```python
from build123d import *

# Parameters (mm, degrees)
BOSS_EXTRUDE1_START             = 3.5
SKETCH1_W                       = 116
SKETCH1_H                       = 42
BOSS_EXTRUDE1_DEPTH             = 3.5
BOSS_EXTRUDE2_REACH             = 64.081
SKETCH2_R                       = 1.75
BOSS_EXTRUDE2_DIRECTION_2_REACH = 64.081
SKETCH2_3_R                     = 1.75
CUT_EXTRUDE1_DEPTH              = 54
BOSS_EXTRUDE3_DEPTH             = 25
BOSS_EXTRUDE5_START             = -4
SKETCH4_R                       = 1.5
BOSS_EXTRUDE5_DEPTH             = 4
SKETCH5_R                       = 1.5
BOSS_EXTRUDE6_DEPTH             = 4
FILLET1_R                       = 5
FILLET2_R                       = 1
SKETCH6_W                       = 116
SKETCH6_H                       = 71
BOSS_EXTRUDE7_DEPTH             = 4
SKETCH7_R                       = 1.5
BOSS_EXTRUDE8_DEPTH             = 4
LPATTERN1_COUNT                 = 2
LPATTERN1_PITCH                 = 112
FILLET3_R                       = 4


with BuildPart() as part:
    # Sketch1 → Boss-Extrude1 (new body)
    with BuildSketch(Plane(origin=(0, 0, 0), x_dir=(1, 0, 0), z_dir=(0, 1, 0)).offset(BOSS_EXTRUDE1_START)):
        Rectangle(SKETCH1_W, SKETCH1_H)
    extrude(amount=BOSS_EXTRUDE1_DEPTH)

    # Boss-Extrude2: up to this face of the body (flat: up to its plane)
    boss_extrude2_end = Plane(part.part.faces().sort_by_distance((58, 5.25, 0))[0])
    # Sketch2 → Boss-Extrude2 (add, up to the picked face)
    with BuildSketch(Plane(origin=(0, 0, 0), x_dir=(0, 0, -1), z_dir=(1, 0, 0)), mode=Mode.PRIVATE) as boss_extrude2_sk1:
        with BuildLine():
            ThreePointArc((10, 13), (8.586149806, 9.094875162), (5, 7))
            Line((5, 7), (10, 7))
            Line((10, 7), (21, 7))
            Line((21, 7), (21, 18))
            Line((21, 18), (15, 18))
            ThreePointArc((15, 18), (11.464466094, 16.535533906), (10, 13))
        make_face()
        with Locations(Location((15.5, 12.475, 0), (0, 0, 180))):
            Circle(SKETCH2_R, mode=Mode.SUBTRACT)
    boss_extrude2_tool1 = split(extrude(boss_extrude2_sk1.sketch, amount=BOSS_EXTRUDE2_REACH, mode=Mode.PRIVATE), bisect_by=boss_extrude2_end, keep=Keep.BOTH, mode=Mode.PRIVATE)
    # Sketch2 → Boss-Extrude2 (add, up to the picked face)
    with BuildSketch(Plane(origin=(0, 0, 0), x_dir=(0, 0, -1), z_dir=(1, 0, 0)), mode=Mode.PRIVATE) as boss_extrude2_sk2:
        with BuildLine():
            Line((-21, 18), (-21, 7))
            Line((-21, 7), (-5, 7))
            ThreePointArc((-5, 7), (-8.586149806, 9.094875162), (-10, 13))
            ThreePointArc((-10, 13), (-11.464466094, 16.535533906), (-15, 18))
            Line((-15, 18), (-21, 18))
        make_face()
        with Locations(Location((-15.5, 12.475, 0), (0, 0, 180))):
            Circle(SKETCH2_R, mode=Mode.SUBTRACT)
    boss_extrude2_tool2 = split(extrude(boss_extrude2_sk2.sketch, amount=BOSS_EXTRUDE2_REACH, mode=Mode.PRIVATE), bisect_by=boss_extrude2_end, keep=Keep.BOTH, mode=Mode.PRIVATE)
    add(boss_extrude2_tool1.solids().sort_by(Axis((0, 8.970574, -8.735311), (1, 0, 0)))[0])
    add(boss_extrude2_tool2.solids().sort_by(Axis((0, 12.5, 20.805835), (1, 0, 0)))[0])

    # Boss-Extrude2 direction 2: up to this face of the body (flat: up to its plane)
    boss_extrude2_direction_2_end = Plane(part.part.faces().sort_by_distance((-58, 5.25, 0))[0])
    # Sketch2 → Boss-Extrude2 direction 2 (add, up to the picked face)
    with BuildSketch(Plane(origin=(0, 0, 0), x_dir=(0, 0, -1), z_dir=(1, 0, 0)), mode=Mode.PRIVATE) as boss_extrude2_direction_2_sk1:
        with BuildLine():
            ThreePointArc((10, 13), (8.586149806, 9.094875162), (5, 7))
            Line((5, 7), (10, 7))
            Line((10, 7), (21, 7))
            Line((21, 7), (21, 18))
            Line((21, 18), (15, 18))
            ThreePointArc((15, 18), (11.464466094, 16.535533906), (10, 13))
        make_face()
        with Locations(Location((15.5, 12.475, 0), (0, 0, 180))):
            Circle(SKETCH2_R, mode=Mode.SUBTRACT)
    boss_extrude2_direction_2_tool1 = split(extrude(boss_extrude2_direction_2_sk1.sketch, amount=-BOSS_EXTRUDE2_DIRECTION_2_REACH, mode=Mode.PRIVATE), bisect_by=boss_extrude2_direction_2_end, keep=Keep.BOTH, mode=Mode.PRIVATE)
    # Sketch2 → Boss-Extrude2 direction 2 (add, up to the picked face)
    with BuildSketch(Plane(origin=(0, 0, 0), x_dir=(0, 0, -1), z_dir=(1, 0, 0)), mode=Mode.PRIVATE) as boss_extrude2_direction_2_sk2:
        with BuildLine():
            Line((-21, 18), (-21, 7))
            Line((-21, 7), (-5, 7))
            ThreePointArc((-5, 7), (-8.586149806, 9.094875162), (-10, 13))
            ThreePointArc((-10, 13), (-11.464466094, 16.535533906), (-15, 18))
            Line((-15, 18), (-21, 18))
        make_face()
        with Locations(Location((-15.5, 12.475, 0), (0, 0, 180))):
            Circle(SKETCH2_R, mode=Mode.SUBTRACT)
    boss_extrude2_direction_2_tool2 = split(extrude(boss_extrude2_direction_2_sk2.sketch, amount=-BOSS_EXTRUDE2_DIRECTION_2_REACH, mode=Mode.PRIVATE), bisect_by=boss_extrude2_direction_2_end, keep=Keep.BOTH, mode=Mode.PRIVATE)
    add(boss_extrude2_direction_2_tool1.solids().sort_by(Axis((0, 8.970574, -8.735311), (-1, 0, 0)))[0])
    add(boss_extrude2_direction_2_tool2.solids().sort_by(Axis((0, 12.5, 20.805835), (-1, 0, 0)))[0])

    # Sketch2<3> → Cut-Extrude1 (cut, symmetric)
    # profile 1 of 2: a face of its own
    with BuildSketch(Plane(origin=(0, 0, 0), x_dir=(0, 0, -1), z_dir=(1, 0, 0))):
        with BuildLine():
            ThreePointArc((10, 13), (8.586149806, 9.094875162), (5, 7))
            Line((5, 7), (10, 7))
            Line((10, 7), (21, 7))
            Line((21, 7), (21, 18))
            Line((21, 18), (15, 18))
            ThreePointArc((15, 18), (11.464466094, 16.535533906), (10, 13))
        make_face()
        with Locations((15.5, 12.475)):
            Circle(SKETCH2_3_R, mode=Mode.SUBTRACT)
    # profile 2 of 2: a face of its own
    with BuildSketch(Plane(origin=(0, 0, 0), x_dir=(0, 0, -1), z_dir=(1, 0, 0))):
        with BuildLine():
            Line((-21, 18), (-21, 7))
            Line((-21, 7), (-5, 7))
            ThreePointArc((-5, 7), (-8.586149806, 9.094875162), (-10, 13))
            ThreePointArc((-10, 13), (-11.464466094, 16.535533906), (-15, 18))
            Line((-15, 18), (-21, 18))
        make_face()
        with Locations((-15.5, 12.475)):
            Circle(SKETCH2_3_R, mode=Mode.SUBTRACT)
    extrude(amount=CUT_EXTRUDE1_DEPTH, both=True, mode=Mode.SUBTRACT)

    # Sketch3 → Boss-Extrude3 (add)
    with BuildSketch(Plane(origin=(-54, 0, 0), x_dir=(0, 0, -1), z_dir=(1, 0, 0))):
        with BuildLine():
            Line((-21, 7), (-15, 7))
            ThreePointArc((-15, 7), (-18.465513805, 9.534486195), (-21, 13))
            Line((-21, 13), (-21, 7))
        make_face()
        with BuildLine():
            Line((21, 7), (21, 13))
            ThreePointArc((21, 13), (18.465513805, 9.534486195), (15, 7))
            Line((15, 7), (21, 7))
        make_face()
    boss_extrude3 = extrude(amount=BOSS_EXTRUDE3_DEPTH)

    # Mirror4: Boss-Extrude3 across plane
    add(boss_extrude3.mirror(Plane(origin=(0, 0, 0), x_dir=(0, 0, 1), z_dir=(1, 0, 0))))

    # Sketch4 → Boss-Extrude5 (add)
    # profile 1 of 2: a face of its own
    with BuildSketch(Plane.ZY.offset(58).offset(BOSS_EXTRUDE5_START)):
        Polygon((21, 18), (35.5, 3.5), (21, 3.5), align=None)
        with Locations((24.5, 7.5)):
            Circle(SKETCH4_R, mode=Mode.SUBTRACT)
    # profile 2 of 2: a face of its own
    with BuildSketch(Plane.ZY.offset(58).offset(BOSS_EXTRUDE5_START)):
        Polygon((-21, 18), (-21, 3.5), (-35.5, 3.5), align=None)
        with Locations(Location((-24.5, 7.5, 0), (0, 0, 180))):
            Circle(SKETCH4_R, mode=Mode.SUBTRACT)
    extrude(amount=BOSS_EXTRUDE5_DEPTH)

    # Sketch5 → Boss-Extrude6 (add)
    # profile 1 of 2: a face of its own
    with BuildSketch(Plane(origin=(58, 0, 0), x_dir=(0, 0, -1), z_dir=(1, 0, 0))):
        Polygon((-35.5, 3.5), (-21, 18), (-21, 3.5), align=None)
        with Locations(Location((-24.5, 7.5, 0), (0, 0, 180))):
            Circle(SKETCH5_R, mode=Mode.SUBTRACT)
    # profile 2 of 2: a face of its own
    with BuildSketch(Plane(origin=(58, 0, 0), x_dir=(0, 0, -1), z_dir=(1, 0, 0))):
        Polygon((21, 18), (21, 3.5), (35.5, 3.5), align=None)
        with Locations((24.5, 7.5)):
            Circle(SKETCH5_R, mode=Mode.SUBTRACT)
    extrude(amount=-BOSS_EXTRUDE6_DEPTH)

    # Fillet1
    fillet1_edges = [part.edges().sort_by_distance(p)[0] for p in [
        (56, 18, -21),
        (56, 18, 21),
        (-56, 18, 21),
        (-56, 18, -21),
    ]]
    fillet(fillet1_edges, radius=FILLET1_R)

    # Fillet2
    fillet2_edges = [part.edges().sort_by_distance(p)[0] for p in [
        (-54, 8.25, 21),
        (-54, 8.25, -21),
        (54, 8.25, 21),
        (54, 8.25, -21),
    ]]
    fillet(fillet2_edges, radius=FILLET2_R)

    # Sketch6 → Boss-Extrude7 (add)
    with BuildSketch(Plane.XZ.offset(-3.5)):
        Rectangle(SKETCH6_W, SKETCH6_H)
    extrude(amount=BOSS_EXTRUDE7_DEPTH)

    # Sketch7 → Boss-Extrude8 (add)
    with BuildSketch(Plane.ZY.offset(58)):
        with BuildLine():
            Line((7.5, -0.5), (-7.5, -0.5))
            ThreePointArc((-7.5, -0.5), (0, -8), (7.5, -0.5))
        make_face()
        with Locations((0, -4)):
            Circle(SKETCH7_R, mode=Mode.SUBTRACT)
    boss_extrude8 = extrude(amount=-BOSS_EXTRUDE8_DEPTH)

    # LPattern1: Boss-Extrude8 ×2
    with Locations(*[(i * LPATTERN1_PITCH, 0, 0) for i in range(1, LPATTERN1_COUNT)]):
        add(boss_extrude8)

    # Fillet3
    fillet3_edges = [part.edges().sort_by_distance(p)[0] for p in [
        (-56, -0.5, 7.5),
        (-56, -0.5, -7.5),
        (56, -0.5, 7.5),
        (56, -0.5, -7.5),
    ]]
    fillet(fillet3_edges, radius=FILLET3_R)


solid = part.part
```
The listing builds one solid part. Answer for the finished solid, in the listing's coordinates (mm). A direction names the side the tool comes from. Give positions to 0.01 mm unless a question says otherwise; leave off trailing zeros. Order: outer loops, then holes, each group sorted by start corner. A loop starts at its lowest first (then second) coordinate and runs counter-clockwise, first axis right, second up.
Item 1: The part is cut by section A-A, the plane z = 24.5. Give the vertices of the cut face in (x, y).
From the geometry:
outline: (-58, -0.5) - (58, -0.5) - (58, 6) - (54, 6) - (54, 3.5) - (-54, 3.5) - (-54, 6) - (-58, 6) - close; (-58, 9) - (-54, 9) - (-54, 14.5) - (-58, 14.5) - close; (54, 9) - (58, 9) - (58, 14.5) - (54, 14.5) - close
Item 2: The part is cut by section C-C, the plane z = -29. Give the vertices of the cut face in (x, y), and give its area (3 significant figures).
From the geometry:
outline: (-58, -0.5) - (58, -0.5) - (58, 10) - (54, 10) - (54, 3.5) - (-54, 3.5) - (-54, 10) - (-58, 10) - close
area: 516 mm2
Item 3: Given pin 1 Ø3.5 at (y, z) = (7.5, 24.5) entering from +X; pin 2 Ø2 at (x, y) = (-15.5, 6.5) entering from -Z; pin 3 Ø2.5 at (y, z) = (-4, 0) entering from +X; pin 4 Ø2 at (x, z) = (6, 9) entering from -Y, each flat-ended and moving along its own axis, determine where each tip first touches the part or whether it passes through.
From the geometry:
pin 1: stops at x = 58
pin 2: stops at z = -21
pin 3: passes through
pin 4: stops at y = -0.5
Item 4: The part is cut by section B-B, the plane x = -27. Give the vertices of the cut face in (y, z), and give its area (3 significant figures).
From the geometry:
outline: (-0.5, -35.5) - (3.5, -35.5) - (3.5, -21) - (7, -21) - (7, 21) - (3.5, 21) - (3.5, 35.5) - (-0.5, 35.5) - close
area: 431 mm2
Item 5: Which of the six approach directions +Z, -Z, +X, -X, +Y, -Y give full straight-line access (tool end or side, diameter ignored) to faces 4 (the face through (-55.97, 9.05, 8.55)), 5 (the face through (-29, 9, 19)), 6 (the face through (-1, 2, -35.5)), 7 (the face through (1, 7, 0))?
From the geometry:
face 4: +X, -X, +Y
face 5: +Z, -Z, +Y
face 6: -Z, +X, -X, +Y, -Y
face 7: +Y
Item 6: For a pull along Y with two mould halves and no side action, classify faces 1 (the face through (-1, 2, 35.5)), 2 (the face through (56.03, 9.05, 8.55)), 3 (the face through (56.028, 13.145, -13.883)) as pulls with the +Y half, pulls with the -Y half, needs draft (parallel to the pull), parting line crosses it, or undercut.
From the geometry:
face 1: needs draft
face 2: pulls with the +Y half
face 3: undercut
Item 7: The part is cut by section D-D, the plane z = 0. Give the vertices of the cut face in (x, y), and give its area (3 significant figures).
From the geometry:
outline: (-58, -8) - (-54, -8) - (-54, -5.5) - (-58, -5.5) - close; (-58, -2.5) - (-54, -2.5) - (-54, -0.5) - (54, -0.5) - (54, -2.5) - (58, -2.5) - (58, 7) - (-58, 7) - close; (54, -8) - (58, -8) - (58, -5.5) - (54, -5.5) - close
area: 906 mm2
Item 8: Find the intervals of material crossed by probe 1 along X at (y, z) = (14.75, -13.5); probe 2 along Y at (x, z) = (-42.5, 11.5); probe 3 along Z at (x, y) = (1, 6.75), in increasing order.
From the geometry:
probe 1: x = -58 to -54, 54 to 58
probe 2: y = -0.5 to 7
probe 3: z = -21 to 21
